Input: part model. Units: mm. Frame: model coordinates. A direction names the side the tool comes from. Coordinates: 2 decimals unless noted, no trailing zeros. Loops run counter-clockwise (first coordinate to the right, second up) from the corner with the lowest first, then second, coordinate; pieces in that order, holes last.
Item 1: Section B-B on x = 20. Return loops of the section in (y, z), and give its area (3 significant figures).
Item 2: Pull-direction query (X, two-part tool) for faces 1 (the cylindrical face through (39.4, 36.94, 0.57)), 2 (the flat face through (20, 6, 6.5)), 3 (the cylindrical face through (27.555, 3.944, 3.87)), 4 (the flat face through (20, 37, 7)); classes: released by +X, released by -X, zero draft, split by the parting line, or undercut.
Item 3: Section A-A on y = 39. Return loops of the section in (x, z).
Item 4: Reachability of faces 5 (the cylindrical face through (22.6, 3.9, 3.5)), 6 (the cylindrical face through (21.615, 2.895, 6.754)), 7 (the cylindrical face through (0.6, 36.94, 6.43)) from +Z, -Z, +X, -X, +Y, -Y: full face, straight path, thin tool, end or side. Return the list, or none.
Item 5: Ray query, line 1 along Z through (x, y) = (17, 7); line 2 along Y through (x, z) = (11, 3.25); line 3 along X through (y, z) = (40, 2.5). Return the intervals inside material, ascending.
Item 6: Contact query for flat-ended pins moving along their axis: P1, Ø1, axis at x = 9, z = 4, coming from the -Y side; P2, Ø1, axis at y = 56, z = 2.5, coming from the +X side; P3, Ø1, axis at x = 5.5, z = 6, coming from the -Y side. Output: stop coordinate, or through.
Item 7: Section C-C on y = 6. Give the number of separate pieces and of enclosed holes in the cut face, and give its area (3 significant figures).
Item 8: Section D-D on x = 29. Return loops of the section in (y, z), and give its area (3 significant figures).
```python
from build123d import *

# Parameters (mm, degrees)
F0_W         = 40
F0_H         = 73
F1_DEPTH     = 7
F3_R         = 1.0007571232
F4_DEPTH     = 8
F6_DEPTH     = 2
F8_DEPTH     = 2.3
F9_R         = 3.5
F10_DEPTH    = 0.5
F11_W        = 12
F11_H        = 1
F12_DEPTH    = 1
F13_T1_DEPTH = 32
F14_R        = 2
F15_R        = 2


# Not quite as in the source:
# - a fillet or chamfer that OpenCascade refuses, or shapes differently, is made with other operations: its cross-section is extruded or revolved along the edge and cut away or added


with BuildPart() as f1:
    # F0 (on Top) → F1 (new body)
    with BuildSketch(Plane.XY):
        with Locations((20, 36.5)):
            Rectangle(F0_W, F0_H)
    extrude(amount=F1_DEPTH)

    # F3 (on face) → F4 (cut)
    with BuildSketch(Plane.XZ):
        with Locations((4.10061609, 3.5689128563)):
            Circle(F3_R)
        with Locations((6.60061609, 3.5689128563)):
            Circle(F3_R)
        with Locations((9.10061609, 3.5689128563)):
            Circle(F3_R)
        with Locations((11.60061609, 3.5689128563)):
            Circle(F3_R)
        with Locations((14.10061609, 3.5689128563)):
            Circle(F3_R)
        with BuildLine():
            Line((21.60061609, 4.5696699795), (16.60061609, 4.5696699795))
            ThreePointArc((16.60061609, 4.5696699795), (15.5998589668, 3.5689128563), (16.60061609, 2.568155733))
            Line((16.60061609, 2.568155733), (21.60061609, 2.568155733))
            ThreePointArc((21.60061609, 2.568155733), (22.6013732132, 3.5689128563), (21.60061609, 4.5696699795))
        make_face()
        with Locations((24.10061609, 3.5689128563)):
            Circle(F3_R)
        with Locations((26.60061609, 3.5689128563)):
            Circle(F3_R)
        with Locations((29.10061609, 3.5689128563)):
            Circle(F3_R)
        with Locations((31.60061609, 3.5689128563)):
            Circle(F3_R)
        with Locations((34.10061609, 3.5689128563)):
            Circle(F3_R)
    extrude(amount=-F4_DEPTH, mode=Mode.SUBTRACT)

    # F5 (on face) → F6 (cut)
    with BuildSketch(Plane.YZ.offset(40)):
        with BuildLine():
            Line((54.2437834144, 4.5), (48.2437834144, 4.5))
            ThreePointArc((48.2437834144, 4.5), (47.2437834144, 3.5), (48.2437834144, 2.5))
            Line((48.2437834144, 2.5), (54.2437834144, 2.5))
            ThreePointArc((54.2437834144, 2.5), (55.2437834144, 3.5), (54.2437834144, 4.5))
        make_face()
    extrude(amount=-F6_DEPTH, mode=Mode.SUBTRACT)

    # F7 (on face) → F8 (join)
    with BuildSketch(Plane.YZ.offset(38)):
        with BuildLine():
            Line((54.2437834144, 4.4), (48.2437834144, 4.4))
            ThreePointArc((48.2437834144, 4.4), (47.3437834144, 3.5), (48.2437834144, 2.6))
            Line((48.2437834144, 2.6), (54.2437834144, 2.6))
            ThreePointArc((54.2437834144, 2.6), (55.1437834144, 3.5), (54.2437834144, 4.4))
        make_face()
    extrude(amount=F8_DEPTH)

    # F9 (on face) → F10 (cut)
    with BuildSketch(Plane.XY.offset(7)):
        with Locations((20, 6)):
            Circle(F9_R)
    extrude(amount=-F10_DEPTH, mode=Mode.SUBTRACT)

    # F11 (on face) → F12 (cut)
    with BuildSketch(Plane.XY.offset(7)):
        with Locations((20, 69.5)):
            Rectangle(F11_W, F11_H)
        with BuildLine():
            ThreePointArc((10.5, 69.5), (10.3535533906, 69.8535533906), (10, 70))
            Line((10, 70), (10, 69))
            ThreePointArc((10, 69), (10.3535533906, 69.1464466094), (10.5, 69.5))
        make_face()
        with BuildLine():
            Line((10, 69), (10, 70))
            ThreePointArc((10, 70), (9.5, 69.5), (10, 69))
        make_face()
    extrude(amount=-F12_DEPTH, mode=Mode.SUBTRACT)

    # F13: fillet of radius 5 on 4 edges, made by hand

    # F13_s2 → F13_t1 (cut)
    with BuildSketch(Plane.XY.offset(-12.5)):
        with BuildLine():
            ThreePointArc((35, 0), (38.5355339059, 1.4644660941), (40, 5))
            Line((40, 5), (40, 0))
            Line((40, 0), (35, 0))
        make_face()
        with BuildLine():
            ThreePointArc((0, 5), (1.4644660941, 1.4644660941), (5, 0))
            Line((5, 0), (0, 0))
            Line((0, 0), (0, 5))
        make_face()
        with BuildLine():
            ThreePointArc((35, 73), (38.5355339059, 71.5355339059), (40, 68))
            Line((40, 68), (40, 73))
            Line((40, 73), (35, 73))
        make_face()
        with BuildLine():
            ThreePointArc((0, 68), (1.4644660941, 71.5355339059), (5, 73))
            Line((5, 73), (0, 73))
            Line((0, 73), (0, 68))
        make_face()
    extrude(amount=F13_T1_DEPTH, mode=Mode.SUBTRACT)

    # F14
    f14_edges = [f1.edges().sort_by_distance(p)[0] for p in [
        (38.535534, 71.535534, 7),
        (20, 73, 7),
        (1.464466, 71.535534, 7),
        (0, 36.5, 7),
        (1.464466, 1.464466, 7),
        (20, 0, 7),
        (38.535534, 1.464466, 7),
        (40, 36.5, 7),
    ]]
    fillet(f14_edges, radius=F14_R)

    # F15
    f15_edges = [f1.edges().sort_by_distance(p)[0] for p in [
        (40, 36.5, 0),
        (38.535534, 71.535534, 0),
        (20, 73, 0),
        (1.464466, 71.535534, 0),
        (0, 36.5, 0),
        (38.535534, 1.464466, 0),
        (20, 0, 0),
        (1.464466, 1.464466, 0),
    ]]
    fillet(f15_edges, radius=F15_R)


solid = f1.part
```
Results found:
1. outline: (0, 2) arc R2 ccw to (2, 0) - (71, 0) arc R2 ccw to (73, 2) - (73, 5) arc R2 ccw to (71, 7) - (70, 7) - (70, 6) - (69, 6) - (69, 7) - (9.5, 7) - (9.5, 6.5) - (2.5, 6.5) - (2.5, 7) - (2, 7) arc R2 ccw to (0, 5) - (0, 4.57) - (8, 4.57) - (8, 2.57) - (0, 2.57) - close
1. area: 487 mm2
2. face 1: released by +X
2. face 2: undercut
2. face 3: undercut
2. face 4: zero draft
3. outline: (0, 2) arc R2 ccw to (2, 0) - (38, 0) arc R2 ccw to (40, 2) - (40, 5) arc R2 ccw to (38, 7) - (2, 7) arc R2 ccw to (0, 5) - close
4. face 5: -Y
4. face 6: +Z
4. face 7: +Z, -X, +Y, -Y
5. line 1: z = 0 to 2.57, 4.57 to 6.5
5. line 2: y = 8 to 73
5. line 3: x = 0 to 40
6. P1: stops at y = 8
6. P2: stops at x = 40
6. P3: stops at y = 0.06
7. separate pieces: 1
7. enclosed holes: 11
7. area: 228 mm2
8. outline: (0, 2) arc R2 ccw to (2, 0) - (71, 0) arc R2 ccw to (73, 2) - (73, 5) arc R2 ccw to (71, 7) - (2, 7) arc R2 ccw to (0, 5) - (0, 4.56) - (8, 4.56) - (8, 2.57) - (0, 2.57) - close
8. area: 492 mm2
